from build123d import *

# Parameters (mm, degrees)
SKETCH1_R           = 50
SKETCH1_R_2         = 2.75
SKETCH1_R_3         = 37
BOSS_EXTRUDE1_DEPTH = 5
SKETCH2_R           = 125
SKETCH2_R_2         = 75
BOSS_EXTRUDE2_DEPTH = 5
FILLET1_R           = 10
SKETCH4_W           = 50
SKETCH4_H           = 20
CUT_EXTRUDE1_DEPTH  = 186.135085845


with BuildPart() as part:
    # Sketch1 → Boss-Extrude1 (new body)
    with BuildSketch(Plane(origin=(0, 0, 0), x_dir=(1, 0, 0), z_dir=(0, 1, 0))):
        with Locations(Location((0, 0, 0), (0, 0, 270))):
            Circle(SKETCH1_R)
        with Locations(Location((0, 44, 0), (0, 0, 270))):
            Circle(SKETCH1_R_2, mode=Mode.SUBTRACT)
        with Locations(Location((38.105117767, -22, 0), (0, 0, 270))):
            Circle(SKETCH1_R_2, mode=Mode.SUBTRACT)
        with Locations(Location((-38.105117767, -22, 0), (0, 0, 270))):
            Circle(SKETCH1_R_2, mode=Mode.SUBTRACT)
        with Locations(Location((0, 0, 0), (0, 0, 270))):
            Circle(SKETCH1_R_3, mode=Mode.SUBTRACT)
    extrude(amount=BOSS_EXTRUDE1_DEPTH)



with BuildPart() as body_2:
    # Sketch2 → Boss-Extrude2 (new body)
    with BuildSketch(Plane(origin=(0, -55, 0), x_dir=(1, 0, 0), z_dir=(0, 1, 0))):
        with Locations(Location((0, 0, 0), (0, 0, 270))):
            Circle(SKETCH2_R)
        with Locations(Location((0, 0, 0), (0, 0, 270))):
            Circle(SKETCH2_R_2, mode=Mode.SUBTRACT)
    extrude(amount=BOSS_EXTRUDE2_DEPTH)


with BuildPart() as part_1:
    add(part.part)

    add(body_2.part)  # Revolve1 merges body 2
    # Sketch3 → Revolve1 (revolve)
    with BuildSketch(Plane.XY, mode=Mode.PRIVATE) as revolve1_sk:
        Polygon((-50, 0), (-75, -50), (-77.5, -50), (-50, 5), align=None)
    revolve(revolve1_sk.sketch.rotate(Axis((0, 0, 0), (0, -1, 0)), 270), axis=Axis((0, 0, 0), (0, -1, 0)))

    # Fillet1
    fillet1_edges = [part_1.edges().sort_by_distance(p)[0] for p in [
        (0, -50, -75),
        (0, -50, -77.5),
    ]]
    fillet(fillet1_edges, radius=FILLET1_R)

    # Sketch4 → Cut-Extrude1 (cut, through all)
    with BuildSketch(Plane.XY):
        with Locations((0, -40)):
            Rectangle(SKETCH4_W, SKETCH4_H)
    extrude(amount=-CUT_EXTRUDE1_DEPTH, mode=Mode.SUBTRACT)


solid = part_1.part
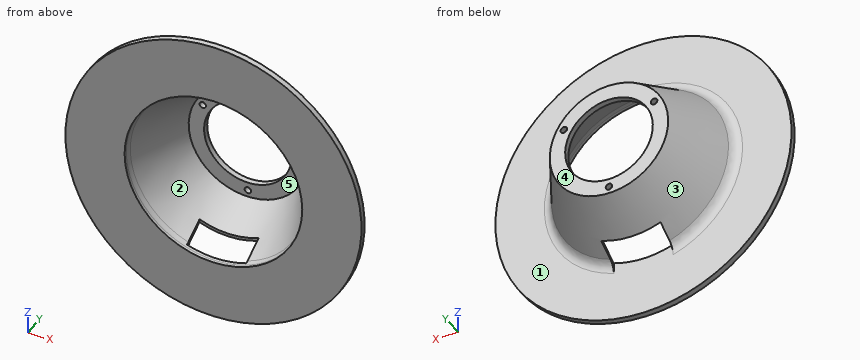
Could you check a few things on this model? Use its own coordinates, in mm. Face numbers are marked on the shaded views. A direction names the side the tool comes from. Give positions to 0.01 mm unless a question says otherwise; leave off trailing zeros. Order: outer loops, then holes, each group sorted by start corner. A loop starts at its lowest first (then second) coordinate and runs counter-clockwise, first axis right, second up.
1. I need wall thicknesses on L1, parallel to X at y = -53.55, z = 0; L2, parallel to Y at x = -80, z = 22.5; L3, parallel to Y at x = 41, z = -20.5. Which ranges of each line are inside material? Lowest first, please.
2. Suppose I cut it at B-B (z = -100). List the corners of the cut face in (x, y) for me.
3. Will these pins go through, and if not, where does the flat tip stop? P1, Ø12, axis at x = -66, y = -27, coming from the +Z side; P2, Ø2.5, axis at x = 5.5, z = -65.5, coming from the -Y side; P3, Ø9, axis at x = -38.11, z = 22, coming from the -Y side.
4. Suppose I cut it at A-A (y = -25). List the corners of the cut face in (x, z) for me, plus the area to 3 significant figures.
5. Suppose I cut it at D-D (x = -102). List the corners of the cut face in (y, z) for me, plus the area to 3 significant figures.
6. We'd pull the mould along Z, two halves only. Please class the marked faces 1, 2 and 3: pulls with the +Z half, pulls with the -Z half, needs draft (parallel to the pull), parting line crosses it, or undercut.
7. For the marked faces 4 and 5, which set-ups out of +Z, -Z, +X, -X, +Y, -Y let a thin tool reach every point of the face, with its end or its side?
8. Suppose I cut it at C-C (x = 6). Give the number of separate pieces and of enclosed holes in the cut face, plus the area to 3 significant figures.
Solved:
1. L1: x = -125 to -75, 75 to 125
1. L2: y = -55 to -49.98
1. L3: y = 0 to 5
2. outline: (-75, -55) - (75, -55) - (75, -50) - (-75, -50) - close
3. P1: stops at z = 29.31
3. P2: stops at y = -30
3. P3: stops at y = 0
4. outline: circle Ø130 at (0, 0); hole circle Ø125 at (0, 0)
4. area: 1,000 mm2
5. outline: (-55, -72.26) - (-50, -72.26) - (-50, 72.26) - (-55, 72.26) - close
5. area: 723 mm2
6. face 1: needs draft
6. face 2: undercut
6. face 3: parting line crosses it
7. face 4: +Z, -Z, +X, -X, +Y
7. face 5: -Y
8. separate pieces: 3
8. enclosed holes: 0
8. area: 853 mm2
